Input: dimensioned drawing with shaded views. Units: mm. Origin: part minimum x, y, z. A direction names the side the tool comes from. Round coordinates to 2 decimals unless told otherwise and drop trailing zeros. Write each loop counter-clockwise with the first axis right and the second up, starting at its lowest first coordinate (ties: lowest second). Pieces come first, ordered by that corner, then holes. Notation, with made-up numbers: (61, 43.5) - (86, 43.5) arc R12 cw to (86, 60.5) - close; hole circle Ø10 at (88.25, 66). An arc over 180 degrees is marked (long way). Use one line per item in the form item = value.
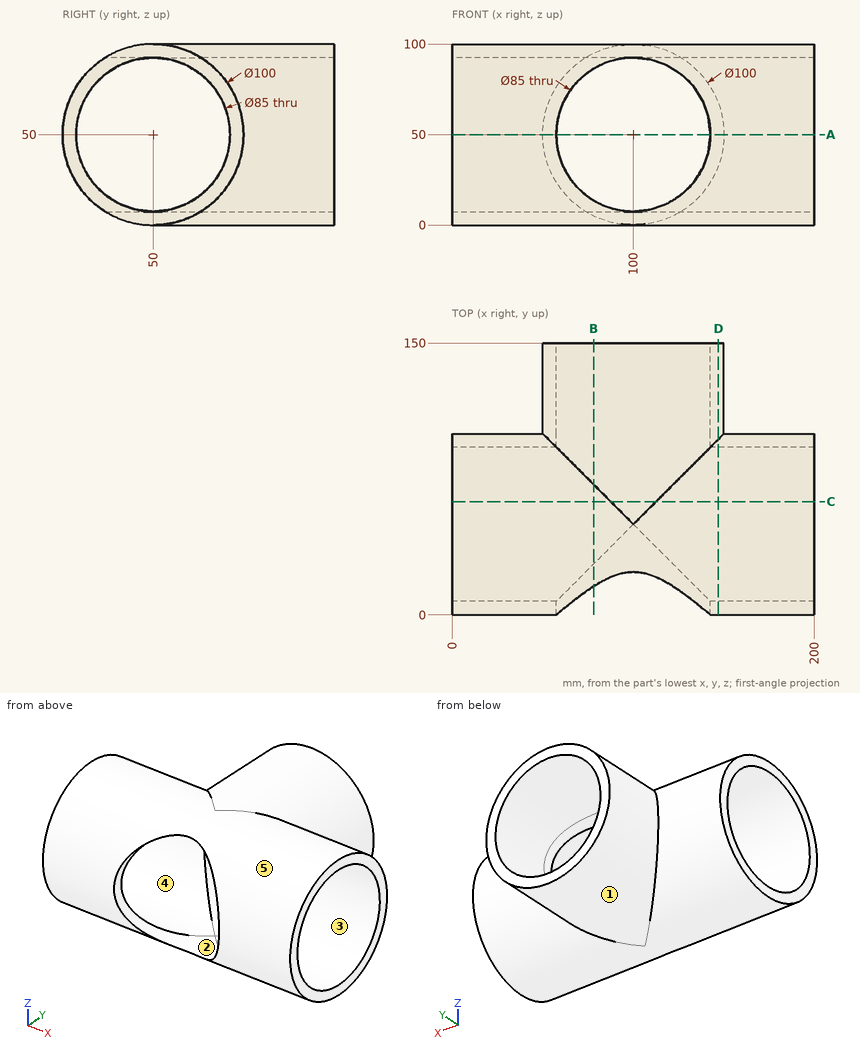
(1) Cut plane A-A on z = 50. Output: boundary loops of the cut face in (x, y).
Derived:
outline = (0, 0) - (57.5, 0) - (57.5, 7.5) - (0, 7.5) - close; (0, 92.5) - (57.5, 92.5) - (57.5, 150) - (50, 150) - (50, 100) - (0, 100) - close; (142.5, 0) - (200, 0) - (200, 7.5) - (142.5, 7.5) - close; (142.5, 92.5) - (200, 92.5) - (200, 100) - (150, 100) - (150, 150) - (142.5, 150) - close
(2) Cut plane C-C on y = 62.5. Output: boundary loops of the cut face in (x, z), then the cut area to 3 significant figures.
Derived:
outline = (0, 1.59) - (87.5, 1.59) arc R50 ccw to (112.5, 1.59) - (200, 1.59) - (200, 9.38) - (112.5, 9.38) arc R42.5 cw to (87.5, 9.38) - (0, 9.38) - close; (0, 90.62) - (87.5, 90.62) arc R42.5 cw to (112.5, 90.62) - (200, 90.62) - (200, 98.41) - (112.5, 98.41) arc R50 ccw to (87.5, 98.41) - (0, 98.41) - close
area = 3,110 mm^2
(3) First-contact query: pin 1 Ø4 at (x, z) = (158, 70) entering from +Y; pin 2 Ø4 at (x, y) = (71.5, 127) entering from +Z; pin 3 Ø1 at (y, z) = (18.5, 75.5) entering from +X; pin 4 Ø12 at (x, z) = (133, 69.5) entering from -Y. Flat tips, straight axial feed; report the tip coordinate or a pass-through.
Derived:
pin_1 = 96.65
pin_2 = 92.4
pin_3 = through
pin_4 = 3.2
(4) Access query for the marked faces 4 and 5. Directions: +Z, -Z, +X, -X, +Y, -Y. A direction counts if a zero-diameter tool reaches every point of the face in a straight line with its end or side. Return the directions, or none.
Derived:
face_4 = +X, -X
face_5 = none
(5) Material intervals for L1, parallel to X at y = 102, z = 50; L2, parallel to Y at x = 167, z = 50; L3, parallel to X at y = 123, z = 61 (3 decimals), sorted ascending.
Derived:
L1 = 50 to 57.5, 142.5 to 150
L2 = 0 to 7.5, 92.5 to 100
L3 = 51.225 to 58.948, 141.052 to 148.775
(6) Draft query along X for the marked faces 1, 2 and 3. Return one class per face: released by +X, released by -X, zero draft, split by the parting line, or undercut.
Derived:
face_1 = split by the parting line
face_2 = undercut
face_3 = zero draft
(7) Cut plane B-B on x = 78. Output: boundary loops of the cut face in (y, z), then the cut area to 3 significant figures.
Derived:
outline = (15.68, 13.64) arc R50 ccw to (72, 5.1) - (150, 5.1) - (150, 13.64) - (72, 13.64) arc R42.5 cw to (28, 13.64) - close; (15.68, 86.36) - (28, 86.36) arc R42.5 cw to (72, 86.36) - (150, 86.36) - (150, 94.9) - (72, 94.9) arc R50 ccw to start
area = 2,140 mm^2
(8) Cut plane D-D on x = 147. Output: boundary loops of the cut face in (y, z), then the cut area to 3 significant figures.
Derived:
outline = (97, 32.94) - (150, 32.94) - (150, 67.06) - (97, 67.06) arc R50 ccw (long way) to start; hole circle Ø85 at (50, 50)
area = 3,920 mm^2
